Can you work these out from the model? Positions are in its coordinate system, mm. A direction names the side the tool comes from. Round coordinates to 2 decimals unless told otherwise and drop trailing zeros. Order: outer loops, then holes, each group sorted by start corner. A loop starts at its lowest first (then second) coordinate and runs counter-clockwise, first axis right, second up. Notation, with made-up numbers: M 82,-2.5 L 106,-2.5 A22 ccw 106,35.5 Z; hole C 20.25,19 d10. An arc over 180 degrees is marked long. Answer as a JSON object with one key per item and string values. Group by question number.
```python
from build123d import *

# Parameters (mm, degrees)
BASE_EXTRUSION_DEPTH = 50
FRONT_CUT_DEPTH      = 20
FRONT_CUT_TAPER      = 10
BACK_CUT_DEPTH       = 20
BACK_CUT_TAPER       = 10
TOP_CUT_SKETCH_R     = 17.5
TOP_CUT_DEPTH        = 50


with BuildPart() as part:
    # Base Sketch → Base Extrusion (new body)
    with BuildSketch(Plane.XY):
        Polygon((0, 0), (0, 50), (75, 50), (75, 100), (100, 100), (100, 25), (125, 25), (125, 0), align=None)
    extrude(amount=BASE_EXTRUSION_DEPTH)

    # Front Cut Sketch → Front Cut (cut)
    with BuildSketch(Plane.XY.offset(50)):
        with BuildLine():
            ThreePointArc((20, 35), (10, 25), (20, 15))
            Line((20, 15), (55, 15))
            ThreePointArc((55, 15), (65, 25), (55, 35))
            Line((55, 35), (20, 35))
        make_face()
    extrude(amount=-FRONT_CUT_DEPTH, taper=FRONT_CUT_TAPER, mode=Mode.SUBTRACT)

    # Back Cut Sketch → Back Cut (cut)
    with BuildSketch(Plane(origin=(0, 0, 0), x_dir=(-1, 0, 0), z_dir=(0, 0, -1))):
        with BuildLine():
            ThreePointArc((-20, 15), (-10, 25), (-20, 35))
            Line((-20, 35), (-55, 35))
            ThreePointArc((-55, 35), (-65, 25), (-55, 15))
            Line((-55, 15), (-20, 15))
        make_face()
    extrude(amount=-BACK_CUT_DEPTH, taper=BACK_CUT_TAPER, mode=Mode.SUBTRACT)

    # Top Cut Sketch → Top Cut (cut)
    with BuildSketch(Plane(origin=(0, 50, 0), x_dir=(1, 0, 0), z_dir=(0, 1, 0))):
        with Locations((37.5, -25)):
            Circle(TOP_CUT_SKETCH_R)
    extrude(amount=-TOP_CUT_DEPTH, mode=Mode.SUBTRACT)


solid = part.part
```
1) Which directions (+Z, -Z, +X, -X, +Y, -Y) give clear straight access to the entire face, cutting with the end or side of a thin tool? Please do faces 4 (the face through (63.21, 25.18, 10.14)), 5 (the face through (20, 50, 19)), 6 (the face through (100, 63, 25)), 7 (the face through (57, 25, 30)), 8 (the face through (0, 25, 25)).
2) I need wall thicknesses on line 1 along Z through (x, y) = (37.5, 12); line 2 along X through (y, z) = (33, 25); line 3 along X through (y, z) = (13, 25). Which ranges of each line are inside material? Lowest first, please.
3) If we section it at B-B on x = 38.5: Write out the boundary of the cut face in (y, z), plus the area to 3 significant figures.
4) If we section it at C-C on y = 46: Write out the boundary of the cut face in (x, z), plus the area to 3 significant figures.
5) For pin 1 (1.5 mm diameter, centred on y = 84, z = 34.5, fed in from +X); pin 2 (7.5 mm diameter, centred on x = 112, z = 19, fed in from +Y); pin 3 (3.5 mm diameter, centred on x = 18, y = 24, fed in from +Z), each with a flat end and sliding along its axis, tell me the tip position at first contact or that it passes through.
6) If we section it at D-D on z = 3: Write out the boundary of the cut face in (x, y), plus the area to 3 significant figures.
7) If we section it at A-A on z = 25: Write out the boundary of the cut face in (x, y), plus the area to 4 significant figures.
8) We'd pull the mould along Y, two halves only. Please class faces 1 (the face through (18, 25, 20)), 2 (the face through (112, 25, 25)), 3 (the face through (63, 0, 25)): +Y half, -Y half, draft (parallel to the pull), parting line (faces both ways), or undercut.
Findings:
{
 "1": {"face 4": "-Z", "face 5": "+Z, -Z, -X, +Y", "face 6": "+Z, -Z, +X, +Y", "face 7": "+Z", "face 8": "+Z, -Z, -X, +Y, -Y"},
 "2": {"line 1": "z = 0 to 7.5, 42.5 to 50", "line 2": "x = 0 to 20, 55 to 100", "line 3": "x = 0 to 20, 55 to 125"},
 "3": {"outline": "M 0,0 L 15,0 L 16.33,7.53 L 0,7.53 Z; M 0,42.47 L 16.33,42.47 L 15,50 L 0,50 Z; M 33.67,7.53 L 35,0 L 50,0 L 50,7.53 Z; M 33.67,42.47 L 50,42.47 L 50,50 L 35,50 Z", "area": "472 mm^2"},
 "4": {"outline": "M 0,0 L 100,0 L 100,50 L 0,50 Z; hole C 37.5,25 d35", "area": "4,040 mm^2"},
 "5": {"pin 1": "stops at x = 100", "pin 2": "stops at y = 25", "pin 3": "stops at z = 30"},
 "6": {"outline": "M 0,0 L 125,0 L 125,25 L 100,25 L 100,100 L 75,100 L 75,50 L 0,50 Z; hole M 20,15.53 L 55,15.53 A9.47 ccw 55,34.47 L 20,34.47 A9.47 ccw Z", "area": "5,930 mm^2"},
 "7": {"outline": "M 0,0 L 20,0 L 20,50 L 0,50 Z; M 55,0 L 125,0 L 125,25 L 100,25 L 100,100 L 75,100 L 75,50 L 55,50 Z", "area": "5,125 mm^2"},
 "8": {"face 1": "undercut", "face 2": "+Y half", "face 3": "-Y half"}
}
